The listing builds one solid part. Answer for the finished solid, in the listing's coordinates (mm). A direction names the side the tool comes from. Round coordinates to 2 decimals unless told otherwise and drop trailing zeros. Order: outer loops, then holes, each group sorted by start corner. A loop starts at its lowest first (then second) coordinate and runs counter-clockwise, first axis right, second up. Notation, with made-up numbers: (48.5, -21) - (68.5, -21) arc R7 ccw to (68.5, -12) - close; hole circle Ø6 at (38, -6.5). An arc over 180 degrees is marked (long way). Write item = value, one per line.
from build123d import *

# Parameters (mm, degrees)
BOSS_EXTRUDE1_DEPTH     = 7.5
SKETCH2_R               = 1.65
CUT_EXTRUDE1_DEPTH      = 15.420976523
MIRROR2_COPY_1_SKETCH_R = 1.65
MIRROR2_COPY_1_DEPTH    = 15.420976523


with BuildPart() as part:
    # Sketch1 → Boss-Extrude1 (new body)
    with BuildSketch(Plane.XY):
        with BuildLine():
            Line((-12, 0), (-5, 0))
            ThreePointArc((-5, 0), (-4.784761162, 1.451227281), (-4.157575752, 2.777510373))
            Line((-4.157575752, 2.777510373), (-12, 2.777510373))
            Line((-12, 2.777510373), (-12, 0))
        make_face()
        with BuildLine():
            ThreePointArc((-4.157575752, 2.777510373), (-4.784761162, 1.451227281), (-5, 0))
            Line((-5, 0), (-1.95, 0))
            ThreePointArc((-1.95, 0), (-1.378858223, 1.378858223), (0, 1.95))
            Line((0, 1.95), (0, 5))
            ThreePointArc((0, 5), (-2.357164413, 4.409509716), (-4.157575752, 2.777510373))
        make_face()
        with BuildLine():
            Line((1.95, 0), (5, 0))
            ThreePointArc((5, 0), (4.784761162, 1.451227281), (4.157575752, 2.777510373))
            ThreePointArc((4.157575752, 2.777510373), (2.357164413, 4.409509716), (0, 5))
            Line((0, 5), (0, 1.95))
            ThreePointArc((0, 1.95), (1.378858223, 1.378858223), (1.95, 0))
        make_face()
        with BuildLine():
            ThreePointArc((4.157575752, 2.777510373), (4.784761162, 1.451227281), (5, 0))
            Line((5, 0), (12, 0))
            Line((12, 0), (12, 2.777510373))
            Line((12, 2.777510373), (4.157575752, 2.777510373))
        make_face()
    boss_extrude1 = extrude(amount=BOSS_EXTRUDE1_DEPTH)

    # Sketch2 → Cut-Extrude1 (cut, symmetric)
    with BuildSketch(Plane(origin=(0, 2.777510373, 0), x_dir=(1, 0, 0), z_dir=(0, 1, 0))):
        with Locations(Location((-7, -3.75, 0), (0, 0, 270))):
            Circle(SKETCH2_R)
    cut_extrude1 = extrude(amount=CUT_EXTRUDE1_DEPTH, both=True, mode=Mode.SUBTRACT)

    # Mirror1: Cut-Extrude1 across plane
    add(cut_extrude1.mirror(Plane(origin=(0, 0, 0), x_dir=(0, 0, 1), z_dir=(1, 0, 0))), mode=Mode.SUBTRACT)

    # Mirror2: Boss-Extrude1, Cut-Extrude1 across plane
    add(boss_extrude1.mirror(Plane.XY))
    add(cut_extrude1.mirror(Plane.XY), mode=Mode.SUBTRACT)

    # Mirror2 copy 1 sketch → Mirror2 copy 1 (cut, symmetric)
    with BuildSketch(Plane(origin=(0, 2.777510373, 0), x_dir=(-1, 0, 0), z_dir=(0, 1, 0))):
        with Locations(Location((-7, -3.75, 0), (0, 0, 270))):
            Circle(MIRROR2_COPY_1_SKETCH_R)
    extrude(amount=MIRROR2_COPY_1_DEPTH, both=True, mode=Mode.SUBTRACT)


solid = part.part
Q1. Section C-C on y = 2.4 is taken. Determine the outline of the cut face in (x, z), then the cut area to 3 significant figures.
Model answer:
outline = (-12, -7.5) - (12, -7.5) - (12, 7.5) - (-12, 7.5) - close; hole circle Ø3.3 at (-7, -3.75); hole circle Ø3.3 at (-7, 3.75); hole circle Ø3.3 at (7, -3.75); hole circle Ø3.3 at (7, 3.75)
area = 326 mm^2
Q2. Section B-B on z = 3.75 is taken. Determine the outline of the cut face in (x, y).
Model answer:
outline = (-12, 0) - (-8.65, 0) - (-8.65, 2.78) - (-12, 2.78) - close; (-5.35, 0) - (-1.95, 0) arc R1.95 cw to (1.95, 0) - (5.35, 0) - (5.35, 2.78) - (4.16, 2.78) arc R5 ccw to (-4.16, 2.78) - (-5.35, 2.78) - close; (8.65, 0) - (12, 0) - (12, 2.78) - (8.65, 2.78) - close
Q3. Section D-D on y = 0.7 is taken. Determine the outline of the cut face in (x, z), then the cut area to 3 significant figures.
Model answer:
outline = (-12, -7.5) - (-1.82, -7.5) - (-1.82, 7.5) - (-12, 7.5) - close; (1.82, -7.5) - (12, -7.5) - (12, 7.5) - (1.82, 7.5) - close; hole circle Ø3.3 at (-7, -3.75); hole circle Ø3.3 at (-7, 3.75); hole circle Ø3.3 at (7, -3.75); hole circle Ø3.3 at (7, 3.75)
area = 271 mm^2
Q4. Flat-ended cylindrical pins translate along their axes: P1, Ø6.5, axis at x = -7, z = -3.5, coming from the +Y side; P2, Ø2, axis at x = -7, z = 3.75, coming from the +Y side; P3, Ø3, axis at x = -6, y = 3.5, coming from the -Z side; P4, Ø1, axis at x = -9, z = 5, coming from the +Y side. Find the tip coordinate at first contact, or state that the pin passes through.
Model answer:
P1 = 3.31
P2 = through
P3 = -7.5
P4 = 2.78
Q5. Determine the mould class of faces 4 (the face through (0, 3, 7.5)), 5 (the face through (-8.464, 1.408, 4.511)), 6 (the face through (-7, 0, 0)) for opening direction Z: released by +Z, released by -Z, zero draft, split by the parting line, or undercut.
Model answer:
face_4 = released by +Z
face_5 = undercut
face_6 = zero draft
Q6. Section A-A on x = -7 is taken. Determine the outline of the cut face in (y, z), then the cut area to 3 significant figures.
Model answer:
outline = (0, -7.5) - (2.78, -7.5) - (2.78, -5.4) - (0, -5.4) - close; (0, -2.1) - (2.78, -2.1) - (2.78, 2.1) - (0, 2.1) - close; (0, 5.4) - (2.78, 5.4) - (2.78, 7.5) - (0, 7.5) - close
area = 23.3 mm^2
Q7. For faces 1 (the face through (-8, 2.778, 0)), 2 (the face through (7, 0, 0)), 3 (the face through (8, 2.778, 0)), determine the directions among +Z, -Z, +X, -X, +Y, -Y from which every point of the face is accessible in a straight line to the end or side of a thin tool.
Model answer:
face_1 = +Z, -Z, -X, +Y
face_2 = +Z, -Z, +X, -X, -Y
face_3 = +Z, -Z, +X, +Y
Q8. Find the intervals of material crossed by line 1 (X direction, y = 2.05, z = -3.75); line 2 (X direction, y = 1.25, z = -3.75); line 3 (Z direction, x = -5.5, y = 0.95), in increasing order. Write a range as from..to.
Model answer:
line_1 = -12..-8.65, -5.35..5.35, 8.65..12
line_2 = -12..-8.65, -5.35..-1.5, 1.5..5.35, 8.65..12
line_3 = -7.5..-4.44, -3.06..3.06, 4.44..7.5
